from build123d import *

# Parameters (mm, degrees)
BOSS_EXTRUDE1_DEPTH = 17.2
CHAMFER1_SIZE       = 3
CHAMFER2_SIZE       = 2
SKETCH3_R           = 2.5
SKETCH3_R_2         = 3
BOSS_EXTRUDE2_DEPTH = 5
BOSS_EXTRUDE3_START = 17.2
SKETCH5_R           = 3
BOSS_EXTRUDE3_DEPTH = 17.2
BOSS_EXTRUDE4_DEPTH = 22.2
FILLET1_R           = 2
SKETCH8_R           = 3
CUT_EXTRUDE3_DEPTH  = 31
CUT_EXTRUDE4_DEPTH  = 5
SKETCH10_R          = 3
CUT_EXTRUDE5_DEPTH  = 44
FILLET2_R           = 2
CHAMFER3_SIZE       = 2
CUT_EXTRUDE6_DEPTH  = 4
CUT_EXTRUDE7_DEPTH  = 5


with BuildPart() as part:
    # Sketch2 → Boss-Extrude1 (new body)
    with BuildSketch(Plane(origin=(0, 0, 0), x_dir=(1, 0, 0), z_dir=(0, 1, 0))):
        with BuildLine():
            Line((-112, 25), (-112, -25))
            Line((-112, -25), (-72.5, -40))
            Line((-72.5, -40), (-20.615528128, -40))
            ThreePointArc((-20.615528128, -40), (-25.226188309, -37.264452544), (-29.478805946, -34))
            Line((-29.478805946, -34), (-77.032741633, -34))
            Line((-77.032741633, -34), (-108, -22.240281633))
            Line((-108, -22.240281633), (-108, 21))
            Line((-108, 21), (-60, 21))
            ThreePointArc((-60, 21), (-58.246211251, 23.246211251), (-56, 25))
            Line((-56, 25), (-112, 25))
        make_face()
    extrude(amount=BOSS_EXTRUDE1_DEPTH)

    # Chamfer1
    chamfer1_edges = [part.edges().sort_by_distance(p)[0] for p in [
        (-112, 8.6, -25),
    ]]
    chamfer(chamfer1_edges, length=CHAMFER1_SIZE)

    # Chamfer2
    chamfer2_edges = [part.edges().sort_by_distance(p)[0] for p in [
        (-108, 8.6, -21),
    ]]
    chamfer(chamfer2_edges, length=CHAMFER2_SIZE)

    # Sketch3 → Boss-Extrude2 (add)
    with BuildSketch(Plane(origin=(0, 17.2, 0), x_dir=(1, 0, 0), z_dir=(0, 1, 0))):
        with BuildLine():
            Line((-72.5, -40), (-20.615528128, -40))
            Line((-20.615528128, -40), (-10.615528128, -40))
            ThreePointArc((-10.615528128, -40), (-7.396351284, -37.204380582), (-9.713234444, -33.625185154))
            ThreePointArc((-9.713234444, -33.625185154), (-27.972872623, -21.03612125), (-35, 0))
            ThreePointArc((-35, 0), (-36.796084568, 11.067971811), (-42, 21))
            ThreePointArc((-42, 21), (-45.527864045, 23.94427191), (-50, 25))
            Line((-50, 25), (-109, 25))
            Line((-109, 25), (-112, 22))
            Line((-112, 22), (-112, -25))
            Line((-112, -25), (-72.5, -40))
        make_face()
        with Locations(Location((-50, 15, 0), (0, 0, 270))):
            Circle(SKETCH3_R, mode=Mode.SUBTRACT)
        with Locations(Location((-78.5, -30, 0), (0, 0, 270))):
            Circle(SKETCH3_R_2, mode=Mode.SUBTRACT)
        with BuildLine():
            Line((-85, 10), (-65, 10))
            Line((-65, 10), (-65, -10))
            Line((-65, -10), (-85, -10))
            ThreePointArc((-85, -10), (-95, 0), (-85, 10))
        make_face(mode=Mode.SUBTRACT)
    extrude(amount=BOSS_EXTRUDE2_DEPTH)

    # Sketch5 → Boss-Extrude3 (add)
    with BuildSketch(Plane.XZ.offset(-17.2).offset(BOSS_EXTRUDE3_START)):
        with BuildLine():
            Line((-73.5, 30), (-73.5, 34))
            Line((-73.5, 34), (-83.5, 34))
            Line((-83.5, 34), (-83.5, 30))
            ThreePointArc((-83.5, 30), (-78.5, 25), (-73.5, 30))
        make_face()
        with Locations(Location((-78.5, 30, 0), (0, 0, 270))):
            Circle(SKETCH5_R, mode=Mode.SUBTRACT)
    extrude(amount=-BOSS_EXTRUDE3_DEPTH)

    # Sketch7 → Boss-Extrude4 (add)
    with BuildSketch(Plane(origin=(0, 22.2, 0), x_dir=(1, 0, 0), z_dir=(0, 1, 0))):
        with BuildLine():
            Line((-112, 5.05), (-112, -12.95))
            Line((-112, -12.95), (-116, -12.95))
            ThreePointArc((-116, -12.95), (-125, -3.95), (-116, 5.05))
            Line((-116, 5.05), (-112, 5.05))
        make_face()
    extrude(amount=-BOSS_EXTRUDE4_DEPTH)

    # Fillet1
    fillet1_edges = [part.edges().sort_by_distance(p)[0] for p in [
        (-112, 11.1, 12.95),
        (-112, 11.1, -5.05),
    ]]
    fillet(fillet1_edges, radius=FILLET1_R)

    # Sketch8 → Cut-Extrude3 (cut)
    with BuildSketch(Plane(origin=(0, 22.2, 0), x_dir=(1, 0, 0), z_dir=(0, 1, 0))):
        with Locations(Location((-116, -3.95, 0), (0, 0, 270))):
            Circle(SKETCH8_R)
    extrude(amount=-CUT_EXTRUDE3_DEPTH, mode=Mode.SUBTRACT)

    # Sketch9 → Cut-Extrude4 (cut)
    with BuildSketch(Plane(origin=(0, 22.2, 0), x_dir=(1, 0, 0), z_dir=(0, 1, 0))):
        Polygon((-110.074764358, -1.664192501), (-115.016949541, 2.324308339), (-120.942185183, 0.03850084), (-121.925235642, -6.235807499), (-116.983050459, -10.224308339), (-111.057814817, -7.93850084), align=None)
    extrude(amount=-CUT_EXTRUDE4_DEPTH, mode=Mode.SUBTRACT)

    # Sketch10 → Cut-Extrude5 (cut)
    with BuildSketch(Plane.XY.offset(40)):
        with Locations((-37.5, 8)):
            Circle(SKETCH10_R)
    extrude(amount=-CUT_EXTRUDE5_DEPTH, mode=Mode.SUBTRACT)

    # Fillet2
    fillet2_edges = [part.edges().sort_by_distance(p)[0] for p in [
        (-83.5, 8.6, 31.544079101),
        (-73.5, 8.6, 34),
    ]]
    fillet(fillet2_edges, radius=FILLET2_R)

    # Chamfer3
    chamfer3_edges = [part.edges().sort_by_distance(p)[0] for p in [
        (-65, 19.7, 10),
        (-65, 19.7, -10),
    ]]
    chamfer(chamfer3_edges, length=CHAMFER3_SIZE)

    # Sketch11 → Cut-Extrude6 (cut)
    with BuildSketch(Plane(origin=(0, 22.2, 0), x_dir=(1, 0, 0), z_dir=(0, 1, 0))):
        Polygon((-72.726497308, -30), (-75.613248654, -25), (-81.386751346, -25), (-84.273502692, -30), (-81.386751346, -35), (-75.613248654, -35), align=None)
    extrude(amount=-CUT_EXTRUDE6_DEPTH, mode=Mode.SUBTRACT)

    # Sketch12 → Cut-Extrude7 (cut)
    with BuildSketch(Plane(origin=(0, 0, 34), x_dir=(-1, 0, 0), z_dir=(0, 0, -1))):
        Polygon((43.850852961, 8), (40.675426481, 13.5), (34.324573519, 13.5), (31.149147039, 8), (34.324573519, 2.5), (40.675426481, 2.5), align=None)
    extrude(amount=-CUT_EXTRUDE7_DEPTH, mode=Mode.SUBTRACT)


solid = part.part
Geometry check sheet. Reference: the model listing, model coordinates, mm. A direction names the side the tool comes from. Coordinates: 2 decimals unless noted, no trailing zeros. Order: outer loops, then holes, each group sorted by start corner. A loop starts at its lowest first (then second) coordinate and runs counter-clockwise, first axis right, second up. Notation, with made-up numbers: (10.5, 15.5) -> (39.5, 15.5) arc R7 cw to (39.5, 21.5) -> close; hole circle Ø1 at (45, -16). An arc over 180 degrees is marked (long way). Use a Markdown table: item, result. Add a question column.
1. Go/stop test with flat-tipped pins: pin 1 Ø6 at (x, y) = (-44.5, 12.5) entering from -Z; pin 2 Ø1 at (y, z) = (5, 7) entering from -X; pin 3 Ø2.5 at (x, y) = (-79, 19.5) entering from +Z. Record where each tip stops, or that it passes through.
2. Mould release check, pull along X, two halves, no side actions. Record for faces 4 (the face through (-110.573, 19.735, 4.845)), 5 (the face through (-58.27, 8.48, -23.22)), 6 (the face through (-83, 8, -21)): pulls with the +X half, pulls with the -X half, needs draft (parallel to the pull), parting line crosses it, or undercut.
3. Cross-section at B-B (y = 19.75). Give the number of separate pieces and of enclosed holes in the cut face, and give its area (3 significant figures).
4. Cross-section at A-A (x = -69.5). Enter the section's corners in (y, z), and give its area (3 significant figures).
5. Material ranges on L1, parallel to X at y = 19.5, z = 7; L2, parallel to Z at x = -71, y = 13; L3, parallel to X at y = 11.75, z = 17.5, recorded low to high.
6. Set-up check for faces 1 (the face through (-25.16, 8.48, 37.31)), 2 (the face through (-40, 11, 39)), 3 (the face through (-74.15, 20.228, 27.535)): record each of +Z, -Z, +X, -X, +Y, -Y from which the full face is reachable in a straight line by a thin tool's end or side.
7. Cross-section at C-C (z = -15). Enter the section's corners in (x, y).
8. Cross-section at D-D (x = -104.5). Enter the section's corners in (y, z).
Filled sheet:
| question | item | result |
|---|---|---|
| 1 | pin 1 | z = 34 |
| 1 | pin 2 | x = -124.63 |
| 1 | pin 3 | z = 38.01 |
| 2 | face 4 | undercut |
| 2 | face 5 | pulls with the +X half |
| 2 | face 6 | needs draft |
| 3 | separate pieces | 1 |
| 3 | enclosed holes | 4 |
| 3 | area | 4,450 mm2 |
| 4 | outline | (0, -25) -> (22.2, -25) -> (22.2, -10) -> (17.2, -10) -> (17.2, -21) -> (0, -21) -> close; (0, 34) -> (17.2, 34) -> (17.2, 10) -> (22.2, 10) -> (22.2, 40) -> (0, 40) -> close |
| 4 | area | 397 mm2 |
| 5 | L1 | -124.47 to -120.98, -110.91 to -92.14, -65 to -34.29 |
| 5 | L2 | -25 to -21, 34 to 40 |
| 5 | L3 | -112 to -108 |
| 6 | face 1 | -Z, +X, -Y |
| 6 | face 2 | -Z |
| 6 | face 3 | +Y |
| 7 | outline | (-112, 0) -> (-108, 0) -> (-108, 17.2) -> (-52.5, 17.2) -> (-52.5, 22.2) -> (-112, 22.2) -> close; (-47.5, 17.2) -> (-38.38, 17.2) -> (-38.38, 22.2) -> (-47.5, 22.2) -> close |
| 8 | outline | (0, -25) -> (22.2, -25) -> (22.2, 27.85) -> (0, 27.85) -> (0, 23.57) -> (17.2, 23.57) -> (17.2, -21) -> (0, -21) -> close |
